Design review of the part built by this model. Coordinates are the model's own, in mm. A direction names the side the tool comes from. Give positions to 0.01 mm unless a question says otherwise; leave off trailing zeros. Order: outer loops, then holes, each group sorted by start corner. A loop starts at its lowest first (then second) coordinate and runs counter-clockwise, first axis right, second up.
Autodesk Fusion 360 part; units mm, degrees
sketch "スケッチ1" plane through (0, 0, 0) normal (0, 0, 1) x (1, 0, 0)
  circle A0 centre (0, 0) radius 46
  dimension "d1" = 92
extrude "押し出し1" add sketch "スケッチ1" along normal blind 10
sketch "スケッチ2" plane through (0, 0, 10) normal (0, 0, 1) x (-1, 0, 0)
  circle A0 centre (0, 0) radius 46
  circle A1 centre (0, 0) radius 40.75
  dimension "d4" = 81.5
extrude "押し出し2" cut sketch "スケッチ2" against normal blind 5
sketch "スケッチ3" plane through (0, 0, 10) normal (0, 0, 1) x (-1, 0, 0)
  circle A0 centre (0, 0) radius 40.75
  circle A1 centre (0, 0) radius 12.5
  dimension "d7" = 25
extrude "押し出し3" cut sketch "スケッチ3" against normal blind 10 contours A1
fillet "フィレット1" radius 3 1 faces at (34.6155, -2.9063, 0)
1. Take a section at D-D (z = 1.75). State the section outline as (x, y) points.
Recorded:
outline: circle Ø91.45 at (0, 0); hole circle Ø25.55 at (0, 0)
2. Take a section at C-C (z = 6.5). State the section outline as (x, y) points, then the cut area to 3 significant figures.
Recorded:
outline: circle Ø81.5 at (0, 0); hole circle Ø25 at (0, 0)
area: 4,730 mm2
3. For pin 1 (2 mm diameter, centred on y = -20.5, z = 3.5, fed in from -X); pin 2 (3 mm diameter, centred on y = 11, z = 9, fed in from -X); pin 3 (20 mm diameter, centred on x = 0, y = 0, fed in from +Z); pin 4 (6 mm diameter, centred on x = 28.5, z = 7, fed in from -Y), all flat-tipped, find the tip position at first contact; note any pin that passes through.
Recorded:
pin 1: stops at x = -41.66
pin 2: stops at x = -39.63
pin 3: passes through
pin 4: stops at y = -37.77
4. Take a section at A-A (y = 0). State the section outline as (x, z) points.
Recorded:
outline: (-46, 3) arc R3 ccw to (-43, 0) - (-15.5, 0) arc R3 ccw to (-12.5, 3) - (-12.5, 10) - (-40.75, 10) - (-40.75, 5) - (-46, 5) - close; (12.5, 3) arc R3 ccw to (15.5, 0) - (43, 0) arc R3 ccw to (46, 3) - (46, 5) - (40.75, 5) - (40.75, 10) - (12.5, 10) - close
5. Machinability: for faces 1 (the face through (-10, -8, 10)), 2 (the face through (-37.64, 15.61, 7.54)), which of the approach directions +Z, -Z, +X, -X, +Y, -Y give a long, thin tool a straight path to every point of the face, cutting with its end or side? Answer none if there is none.
Recorded:
face 1: +Z, +X, -X, +Y, -Y
face 2: +Z
6. For line 1 along X through (y, z) = (0, 5.75); line 2 along Y through (x, z) = (0, 4.5), list the stretches that pass through material, from the lowest coordinate up.
Recorded:
line 1: x = -40.75 to -12.5, 12.5 to 40.75
line 2: y = -46 to -12.5, 12.5 to 46
